Here's how the part is built. I have some questions about the finished solid (model axes, mm). A direction names the side the tool comes from. Give positions to 0.01 mm unless a question says otherwise; leave off trailing zeros. Order: outer loops, then holes, each group sorted by start corner. A loop starts at its lowest first (then second) coordinate and runs counter-clockwise, first axis right, second up.
from build123d import *
from build123d.topology import SkipClean

# Parameters (mm, degrees)
SKETCH1_W           = 15.24
SKETCH1_H           = 279.4
BOSS_EXTRUDE3_DEPTH = 6.35
SKETCH2_R           = 2.75
CUT_EXTRUDE1_DEPTH  = 174.437553604
CHAMFER1_SIZE       = 3.175


with BuildPart() as part:
    # Sketch1 → Boss-Extrude3 (new body)
    with BuildSketch(Plane.XY.offset(8)):
        with BuildLine():
            Line((-69.85, -152.4), (-44.45, -152.4))
            ThreePointArc((-44.45, -152.4), (-35.469743879, -148.680256121), (-31.75, -139.7))
            Line((-31.75, -139.7), (-31.75, 139.7))
            ThreePointArc((-31.75, 139.7), (-35.469743879, 148.680256121), (-44.45, 152.4))
            Line((-44.45, 152.4), (-69.85, 152.4))
            ThreePointArc((-69.85, 152.4), (-78.830256121, 148.680256121), (-82.55, 139.7))
            Line((-82.55, 139.7), (-82.55, -139.7))
            ThreePointArc((-82.55, -139.7), (-78.830256121, -148.680256121), (-69.85, -152.4))
        make_face()
        with Locations((-57.15, 0)):
            Rectangle(SKETCH1_W, SKETCH1_H, mode=Mode.SUBTRACT)
        with BuildLine():
            ThreePointArc((-44.45, -136.95), (-39.755456352, -135.005456352), (-41.7, -139.7))
            ThreePointArc((-41.7, -139.7), (-42.505456352, -137.755456352), (-44.45, -136.95))
        make_face(mode=Mode.SUBTRACT)
        with BuildLine():
            ThreePointArc((-72.6, -139.7), (-74.544543648, -135.005456352), (-69.85, -136.95))
            ThreePointArc((-69.85, -136.95), (-71.794543648, -137.755456352), (-72.6, -139.7))
        make_face(mode=Mode.SUBTRACT)
        with BuildLine():
            ThreePointArc((-41.7, 139.7), (-39.755456352, 135.005456352), (-44.45, 136.95))
            ThreePointArc((-44.45, 136.95), (-42.505456352, 137.755456352), (-41.7, 139.7))
        make_face(mode=Mode.SUBTRACT)
        with BuildLine():
            ThreePointArc((-69.85, 136.95), (-74.544543648, 135.005456352), (-72.6, 139.7))
            ThreePointArc((-72.6, 139.7), (-71.794543648, 137.755456352), (-69.85, 136.95))
        make_face(mode=Mode.SUBTRACT)
    extrude(amount=-BOSS_EXTRUDE3_DEPTH)

    # Sketch2 → Cut-Extrude1 (cut, through all)
    with SkipClean():  # the faces are left unmerged after this step: merging them gives an invalid solid
        with BuildSketch(Plane.XY.offset(8)):
            with Locations(Location((-41.7, 136.95, 0), (0, 0, 180))):
                Circle(SKETCH2_R)
            with Locations(Location((-72.6, 136.95, 0), (0, 0, 180))):
                Circle(SKETCH2_R)
            with Locations(Location((-41.7, -136.95, 0), (0, 0, 180))):
                Circle(SKETCH2_R)
            with Locations(Location((-72.6, -136.95, 0), (0, 0, 180))):
                Circle(SKETCH2_R)
        extrude(amount=-CUT_EXTRUDE1_DEPTH, mode=Mode.SUBTRACT)

    # Chamfer1
    chamfer1_edges = [part.edges().sort_by_distance(p)[0] for p in [
        (-39.755456352, 135.005456352, 1.65),
        (-72.6, 134.2, 1.65),
        (-72.6, -134.2, 1.65),
    ]]
    chamfer(chamfer1_edges, length=CHAMFER1_SIZE)


solid = part.part
Q1. If we section it at C-C on z = 3.5: List the corners of the cut face in (x, y) for me (3 decimals).
Filled sheet:
outline: (-82.55, -139.7) arc R12.7 ccw to (-69.85, -152.4) - (-44.45, -152.4) arc R12.7 ccw to (-31.75, -139.7) - (-31.75, 139.7) arc R12.7 ccw to (-44.45, 152.4) - (-69.85, 152.4) arc R12.7 ccw to (-82.55, 139.7) - close; hole circle Ø8.15 at (-72.6, -136.95); hole circle Ø8.15 at (-72.6, 136.95); hole (-64.77, -139.7) - (-49.53, -139.7) - (-49.53, 139.7) - (-64.77, 139.7) - close; hole circle Ø8.15 at (-41.7, 136.95); hole circle Ø5.5 at (-41.7, -136.95)
Q2. I need wall thicknesses on L1, parallel to X at y = -136.95, z = 7.4; L2, parallel to X at y = -49.5, z = 4; L3, parallel to Y at x = -72.6, z = 6.2. Which ranges of each line are inside material? Lowest first, please.
Filled sheet:
L1: x = -82.55 to -75.35, -69.85 to -64.77, -49.53 to -44.45, -38.95 to -31.75
L2: x = -82.55 to -64.77, -49.53 to -31.75
L3: y = -152.1 to -139.7, -134.2 to 134.2, 139.7 to 152.1
Q3. For faces 1 (the face through (-57, -152.4, 5)), 2 (the face through (-57, 139.7, 5)), which set-ups out of +Z, -Z, +X, -X, +Y, -Y let a thin tool reach every point of the face, with its end or its side?
Filled sheet:
face 1: +Z, -Z, +X, -X, -Y
face 2: +Z, -Z
Q4. I'm going to push flat-ended pins straight in: P1, Ø6.5, axis at x = -41.7, y = -136.95, coming from the -Z side; P2, Ø9, axis at x = -72.6, y = 136.95, coming from the -Z side (3 decimals). Where does each tip first touch, or does it pass through?
Filled sheet:
P1: stops at z = 1.65
P2: stops at z = 3.075
Q5. If we section it at A-A on y = -51.5: List the corners of the cut face in (x, z) for me.
Filled sheet:
outline: (-82.55, 1.65) - (-64.77, 1.65) - (-64.77, 8) - (-82.55, 8) - close; (-49.53, 1.65) - (-31.75, 1.65) - (-31.75, 8) - (-49.53, 8) - close
Q6. Thinking about a two-plate mould opening in Y: for faces 3 (the face through (-35.57, -148.78, 4.87)), 4 (the face through (-57, -139.7, 5)), 5 (the face through (-82.55, 2, 5)), which applies, released by +Y, released by -Y, zero draft, split by the parting line, or undercut?
Filled sheet:
face 3: released by -Y
face 4: undercut
face 5: zero draft
Q7. If we section it at B-B on x = -57.5: List the corners of the cut face in (y, z) for me, plus the area to 3 significant figures.
Filled sheet:
outline: (-152.4, 1.65) - (-139.7, 1.65) - (-139.7, 8) - (-152.4, 8) - close; (139.7, 1.65) - (152.4, 1.65) - (152.4, 8) - (139.7, 8) - close
area: 161 mm2
